Verification items for the finished model (mm, model axes). A direction names the side the tool comes from. Round coordinates to 2 decimals unless told otherwise and drop trailing zeros. Write each loop counter-clockwise with the first axis right and the second up, starting at its lowest first coordinate (ties: lowest second). Pieces come first, ordered by that corner, then holes. Notation, with made-up numbers: M 19,-25 L 27,-25 A26 ccw 27,-3 Z; hole C 18.5,20.5 d3. An arc over 180 degrees is marked long. One line per question, with ' | ' between items. Start each with the question number.
Q1. Cross-section at D-D (z = -4). Record the boundary of the cut face in (x, y), then the cut area to 3 significant figures.
Q2. Thickness scan on line 1 along Z through (x, y) = (-6.25, -1.75); line 2 along Y through (x, z) = (0.25, 1); line 3 along Z through (x, y) = (-7.75, -6). Record the ranges inside material, lowest first. Write a range as from..to.
Q3. Cross-section at B-B (y = 0). Record the boundary of the cut face in (x, z), then the cut area to 3 significant figures.
Q4. Tool access check on faces 1 (the face through (0, 2.5, -22)), 2 (the face through (0, -2.5, -22)), 3 (the face through (-0.54, 2.44, -9.86)), 4 (the face through (-15, 0, -22)), 5 (the face through (0, 0, 12)). Record the directions out of +Z, -Z, +X, -X, +Y, -Y that give a thin tool (end or side, any length) a straight path to the whole face; none if there is none.
Q5. Cross-section at A-A (x = 5.5). Record the boundary of the cut face in (y, z).
Q6. Gauge pin test, flat ends, axial feed: pin 1 (4 mm diameter, centred on y = -10, z = -0.5, fed in from -X); pin 2 (6 mm diameter, centred on x = 4.5, z = 1.5, fed in from +Y); pin 3 (3.5 mm diameter, centred on x = -6, z = -22, fed in from -Y). Record the tip position at first contact, or that the pin passes through.
Q7. Cross-section at C-C (x = -8.5). Record the boundary of the cut face in (y, z).
Q8. Release check for a two-part mould opening along Z. For faces 6 (the face through (0, -3, 0)), 7 (the face through (15, 0, -22)), 8 (the face through (0, 0, -23.4)), 9 (the face through (9, 0, -20)) record: released by +Z, released by -Z, zero draft, split by the parting line, or undercut.
from build123d import *

# Parameters (mm, degrees)
F0_R     = 12.5
F1_DEPTH = 12
F2_R     = 2.5
F3_DEPTH = 20
F4_W     = 30
F4_H     = 5
F5_DEPTH = 3.4


with BuildPart() as f1:
    # F0 (on Top) → F1 (new body)
    with BuildSketch(Plane.XY):
        Circle(F0_R)
    extrude(amount=F1_DEPTH)

    # F2 (on face) → F3 (join)
    with BuildSketch(Plane(origin=(0, 0, 0), x_dir=(1, 0, 0), z_dir=(0, 0, -1))):
        Circle(F2_R)
    extrude(amount=F3_DEPTH)

    # F4 (on face) → F5 (join)
    with BuildSketch(Plane(origin=(0, 0, -20), x_dir=(1, 0, 0), z_dir=(0, 0, -1))):
        Rectangle(F4_W, F4_H)
    extrude(amount=F5_DEPTH)


solid = f1.part
Determined:
1) outline: C 0,0 d5 | area: 19.6 mm²
2) line 1: z = -23.4..-20, 0..12 | line 2: y = -12.5..12.5 | line 3: z = 0..12
3) outline: M -15,-23.4 L 15,-23.4 L 15,-20 L 2.5,-20 L 2.5,0 L 12.5,0 L 12.5,12 L -12.5,12 L -12.5,0 L -2.5,0 L -2.5,-20 L -15,-20 Z | area: 502 mm²
4) face 1: -Z, +X, -X, +Y | face 2: -Z, +X, -X, -Y | face 3: none | face 4: +Z, -Z, -X, +Y, -Y | face 5: +Z, +X, -X, +Y, -Y
5) outline: M -11.22,0 L 11.22,0 L 11.22,12 L -11.22,12 Z; M -2.5,-23.4 L 2.5,-23.4 L 2.5,-20 L -2.5,-20 Z
6) pin 1: stops at x = -9.55 | pin 2: stops at y = 12.41 | pin 3: stops at y = -2.5
7) outline: M -9.17,0 L 9.17,0 L 9.17,12 L -9.17,12 Z; M -2.5,-23.4 L 2.5,-23.4 L 2.5,-20 L -2.5,-20 Z
8) face 6: undercut | face 7: zero draft | face 8: released by -Z | face 9: undercut
